Could you check a few things on this model? Use its own coordinates, in mm. A direction names the side the tool comes from. Coordinates: 2 decimals unless noted, no trailing zeros. Loops run counter-clockwise (first coordinate to the right, second up) from the corner with the lowest first, then second, coordinate; pieces in that order, holes last. Notation, with made-up numbers: (88.5, -20) -> (141.5, -20) arc R29 cw to (141.5, 16) -> close; hole circle Ø1 at (3.5, 6.25). An arc over 180 degrees is marked (long way). One line per question, with ' | ' between items. Start each with the question number.
(1) Which directions (+Z, -Z, +X, -X, +Y, -Y) give clear straight access to the entire face, cutting with the end or side of a thin tool? Please do faces 1 (the face through (-12.933, -30.968, 17.261)), 2 (the face through (-16.992, -17.514, 19.147)), 3 (the face through (-19, -11, 30)).
(2) Suppose I cut it at C-C (x = -24). Please give me the cut outline in (y, z), plus the area to 3 significant figures.
(3) Suppose I cut it at D-D (y = -22.5). Give the number of separate pieces and of enclosed holes in the cut face, plus the area to 3 significant figures.
(4) If we mould it in two halves opening along Z, with no side actions, what happens to faces 4 (the face through (-19, -11, 0)), 5 (the face through (-23, -10.949, 17)), 6 (the face through (-31.333, -15.3, 14.79))? For each: pulls with the +Z half, pulls with the -Z half, needs draft (parallel to the pull), parting line crosses it, or undercut.
(5) Suppose I cut it at B-B (z = 4.5). Please give me the cut outline in (x, y) (3 decimals).
(6) If I drill on line 1 along X through (y, z) = (-4.5, 4.5) (3 decimals); line 2 along X through (y, z) = (-16.5, 23.25) (3 decimals); line 3 along Y through (x, z) = (-22.5, 1.75), over which ranges is the centre line in solid material (lowest first)?
(7) Suppose I cut it at A-A (z = 15.75). Please give me the cut outline in (x, y) (3 decimals), plus the area to 3 significant figures.
(8) I'm going to push flat-ended pins straight in: pin 1 Ø2 at (x, z) = (-26, 15) entering from +Y; pin 2 Ø10 at (x, z) = (-23.5, 16) entering from -Y; pin 3 Ø8 at (y, z) = (-24.5, 21.5) entering from +X. Where does each tip first touch, or does it pass through?
```python
from build123d import *

# Parameters (mm, degrees)
F1_DEPTH = 30
F2_R     = 7.0607743661
F3_DEPTH = 12.95017
F4_R     = 1.9790251597
F5_ANGLE = 211.8266616901


# Not quite as in the source:
# - a feature of the source that left no trace in its solid (it failed there, or was rolled back) is left out


with BuildPart() as f1:
    # F0 (on Top) → F1 (new body)
    with BuildSketch(Plane.XY):
        with BuildLine():
            Line((-8.5449986998, 1.5012763055), (-22.9009841796, 1.5012763055))
            Line((-22.9009841796, 1.5012763055), (-25.5437633875, -3.7646328319))
            ThreePointArc((-25.5437633875, -3.7646328319), (-25.5119398754, -4.015202253), (-25.5013069136, -4.2675605514))
            ThreePointArc((-25.5013069136, -4.2675605514), (-25.9427272038, -5.8339799934), (-27.1370868258, -6.9394332191))
            Line((-27.1370868258, -6.9394332191), (-35.6483731166, -23.8987236945))
            Line((-35.6483731166, -23.8987236945), (-8.5449986998, -23.8987236945))
            Line((-8.5449986998, -23.8987236945), (-8.5449986998, 1.5012763055))
        make_face()
    extrude(amount=F1_DEPTH)

    # F2 (on face) → F3 (cut)
    with BuildSketch(Plane.XZ.offset(23.8987236945)):
        with Locations((-23.7271394581, 17.0257668942)):
            Circle(F2_R)
    extrude(amount=-F3_DEPTH, mode=Mode.SUBTRACT)

    # F4 (on face) → F5 (revolve)
    with BuildSketch(Plane.YZ.offset(-8.5449986998)):
        with Locations((-15.5504914001, 17.2328893095)):
            Circle(F4_R)
    revolve(axis=Axis((-8.5449986998, -23.8987236945, 15), (0, 0, -1)), revolution_arc=F5_ANGLE)


solid = f1.part
```
Checks:
1) face 1: +Z, -Z, -X | face 2: -Y | face 3: +Z, +X, -X, +Y, -Y
2) outline: (-23.9, 0) -> (-0.69, 0) -> (-0.69, 30) -> (-23.9, 30) -> (-23.9, 24.08) -> (-10.95, 24.08) -> (-10.95, 9.97) -> (-23.9, 9.97) -> close | area: 514 mm^2
3) separate pieces: 2 | enclosed holes: 1 | area: 648 mm^2
4) face 4: pulls with the -Z half | face 5: undercut | face 6: needs draft
5) outline: (-35.648, -23.899) -> (-8.545, -23.899) -> (-8.545, 1.501) -> (-22.901, 1.501) -> (-25.544, -3.765) arc R3 cw to (-27.137, -6.939) -> close
6) line 1: x = -25.51 to -8.545 | line 2: x = -31.935 to -27.061, -20.393 to -8.545 | line 3: y = -23.9 to 1.5
7) outline: (-35.648, -23.899) -> (-30.672, -23.899) -> (-30.672, -13.982) -> close; (-29.149, -10.949) -> (-16.783, -10.949) -> (-16.783, -23.899) -> (-8.545, -23.899) -> (-8.545, -16.861) arc R7.038 cw (long way) to (-12.256, -29.878) -> (-13.639, -32.105) arc R9.659 ccw (long way) to (-8.545, -14.24) -> (-8.545, 1.501) -> (-22.901, 1.501) -> (-25.544, -3.765) arc R3 cw to (-27.137, -6.939) -> close | area: 428 mm^2
8) pin 1: stops at y = -2.68 | pin 2: stops at y = -10.95 | pin 3: stops at x = 1.76
